Check sheet for the modelled part. Datum: model origin and axes. Units: mm. Face numbers are marked on the shaded views. A direction names the side the tool comes from. Coordinates: 2 decimals unless noted, no trailing zeros. Loops run counter-clockwise (first coordinate to the right, second up) from the corner with the lowest first, then second, coordinate; pieces in that order, holes last. Notation, with made-up numbers: (-26, 35) -> (20, 35) arc R14 cw to (20, 45) -> close; hole circle Ø11 at (31, -29). An arc over 180 degrees is marked (long way). Use CSV: the item, a comma, the result in double quotes. Start each with the question number.
1. Sectioned sample at B-B, the plane z = 35.5. Record the cut outline in (x, y), and give its area (3 significant figures).
2. Sectioned sample at C-C, the plane x = -20. Record the cut outline in (y, z), and give its area (3 significant figures).
3. Set-up check for the marked faces 1 and 2: record each of +Z, -Z, +X, -X, +Y, -Y from which the full face is reachable in a straight line by a thin tool's end or side.
4. Sectioned sample at D-D, the plane x = 30. Record the cut outline in (y, z).
5. Gauge pin test, flat ends, axial feed: pin 1 (8 mm diameter, centred on x = 38.5, z = 23.5, fed in from +Y); pin 2 (12 mm diameter, centred on x = 55.5, z = 7, fed in from -Y); pin 3 (0.6 mm diameter, centred on x = -32, z = 30.5, fed in from +Y). Record the tip position at first contact, or that the pin passes through.
6. Release check for a two-part mould opening along X. For the marked faces 3, 4 and 5 record: pulls with the +X half, pulls with the -X half, needs draft (parallel to the pull), parting line crosses it, or undercut.
7. Thickness scan on L1, parallel to X at y = -9, z = 24 (3 decimals); L2, parallel to X at y = -16.5, z = 40.5; L3, parallel to Y at x = 45.5, z = 37.5. Record the ranges inside material, lowest first.
8. Sectioned sample at A-A, the plane y = -21. Record the cut outline in (x, z).
```python
from build123d import *

# Parameters (mm, degrees)
F1_DEPTH = 50.546
F2_R     = 1.27


with BuildPart() as f1:
    # F0 (on Top) → F1 (new body)
    with BuildSketch(Plane.XY):
        Polygon((-31.618166, -32.146781), (-31.618166, 12.303219), (-32.380166, 12.303219), (-32.380166, -34.073195), (10.55717, 11.709783), (50.289296, -33.25828), (94.619834, 11.003976), (94.619834, -32.146781), (95.381834, -32.146781), (95.381834, 12.841604), (50.324047, -32.146781), (10.573965, 12.841604), align=None)
    extrude(amount=F1_DEPTH)

    # F2
    f2_edges = [f1.edges().sort_by_distance(p)[0] for p in [
        (10.55717, 11.709783, 25.273),
        (-31.618166, -32.146781, 25.273),
        (50.324047, -32.146781, 25.273),
        (94.619834, 11.003976, 25.273),
    ]]
    fillet(f2_edges, radius=F2_R)


solid = f1.part
```
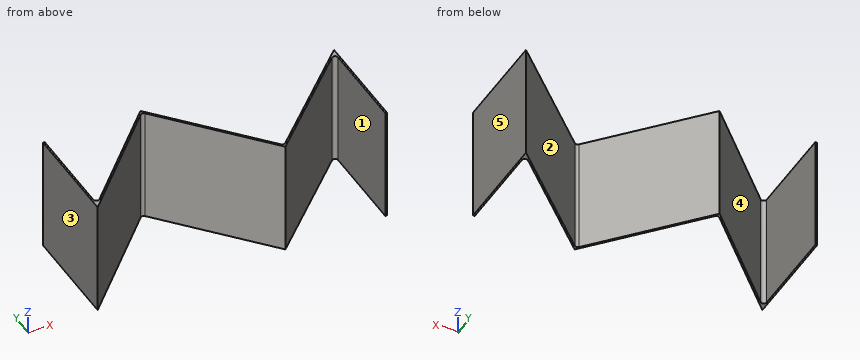
Completed:
1,outline,"(-32.38, -34.07) -> (9.6, 10.69) arc R1.27 cw to (11.48, 10.66) -> (50.29, -33.26) -> (92.45, 8.84) arc R1.27 cw to (94.62, 7.94) -> (94.62, -32.15) -> (95.38, -32.15) -> (95.38, 12.84) -> (51.28, -31.19) arc R1.27 cw to (49.43, -31.14) -> (10.57, 12.84) -> (-29.42, -29.8) arc R1.27 cw to (-31.62, -28.94) -> (-31.62, 12.3) -> (-32.38, 12.3) -> close"
1,area,"214 mm²"
2,outline,"(-20.87, 0) -> (-19.76, 0) -> (-19.76, 50.55) -> (-20.87, 50.55) -> close"
2,area,"56.3 mm²"
3,face 1,"+Z, -Z, -Y"
3,face 2,"+Z, -Z, +Y"
4,outline,"(-10.3, 0) -> (-9.14, 0) -> (-9.14, 50.55) -> (-10.3, 50.55) -> close"
5,pin 1,"y = -14.24"
5,pin 2,"y = -33.26"
5,pin 3,"y = 12.3"
6,face 3,"pulls with the -X half"
6,face 4,"undercut"
6,face 5,"pulls with the +X half"
7,L1,"-32.38 to -31.618, -9.91 to -8.865, 28.856 to 29.872, 73.507 to 74.585, 94.62 to 95.382"
7,L2,"-32.38 to -31.62, -16.94 to -15.9, 35.48 to 36.5, 65.99 to 67.07, 94.62 to 95.38"
7,L3,"-27.84 to -26.69"
8,outline,"(-32.38, 0) -> (-31.62, 0) -> (-31.62, 50.55) -> (-32.38, 50.55) -> close; (-21.16, 0) -> (-20.12, 0) -> (-20.12, 50.55) -> (-21.16, 50.55) -> close; (39.46, 0) -> (40.48, 0) -> (40.48, 50.55) -> (39.46, 50.55) -> close; (61.49, 0) -> (62.57, 0) -> (62.57, 50.55) -> (61.49, 50.55) -> close; (94.62, 0) -> (95.38, 0) -> (95.38, 50.55) -> (94.62, 50.55) -> close"
